Job drawing, mm, ordinate dimensions from the low corner. One solid piece. A direction names the side the tool comes from. Coordinates: 2 decimals unless noted, no trailing zeros. Write each loop counter-clockwise with the first axis right and the second up, starting at its lowest first coordinate (ties: lowest second). Pieces come first, ordered by that corner, then holes. Notation, with made-up numbers: (29, 43) - (83, 43) arc R12 cw to (83, 52) - close; hole circle Ø4 at (-16, 42). An arc over 180 degrees is marked (long way). Use one line per item in the form item = value. Start each with the question number.
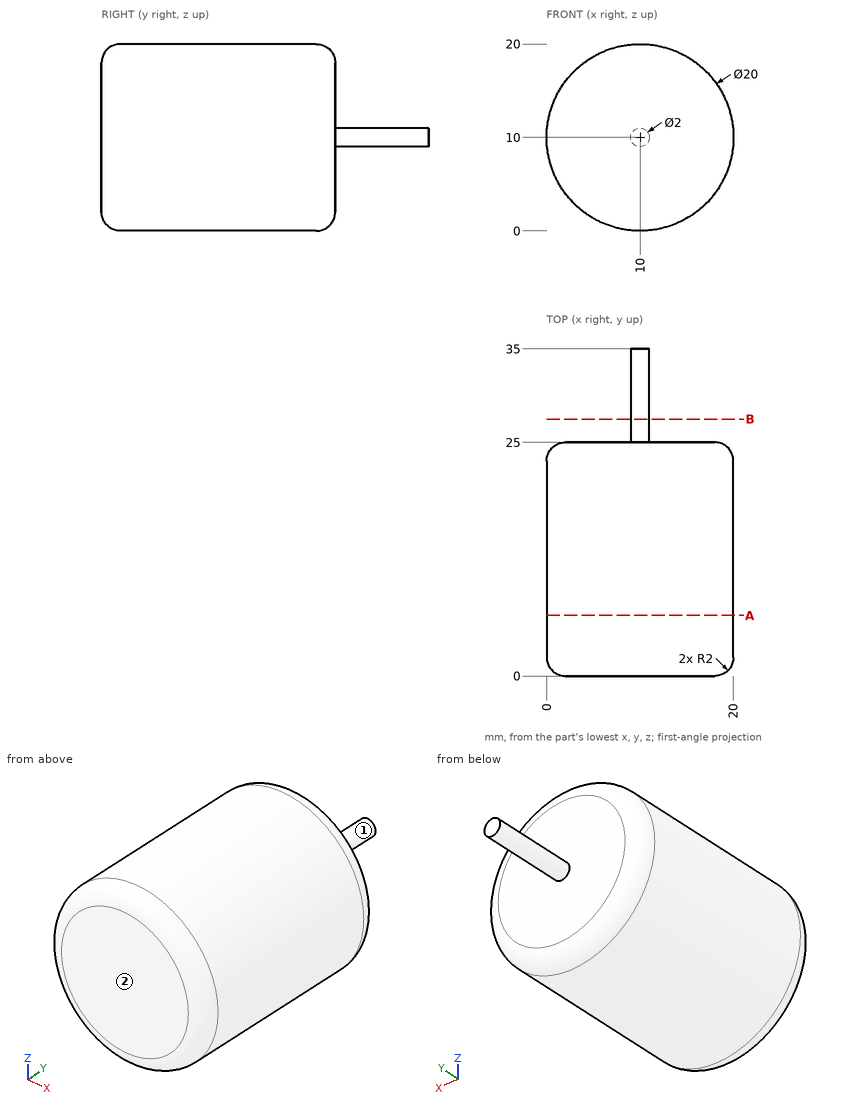
Q1. Which spindle directions (+Z, -Z, +X, -X, +Y, -Y) get a long thin tool onto all of the face, cutting with end or side? Do the marked faces 1 and 2. Say none if no direction does.
Q2. Pin check, flat tips, straight feed: P1, Ø12, axis at y = 15, z = 16.5, coming from the +X side; P2, Ø1.5, axis at x = 7.5, z = 7, coming from the +Y side; P3, Ø3, axis at y = 21.5, z = 5.5, coming from the -X side. Stop position of each tip, or through.
Q3. Drill centre lines: probe 1 along Y at (x, z) = (15, 4.25); probe 2 along X at (y, z) = (17, 16); probe 3 along Z at (x, y) = (10.25, 8.5). Where is each one in solid material? Low to high.
Q4. Slice it at A-A (y = 6.5). List the corners of the cut face in (x, z), plus the area to 3 significant figures.
Q5. Slice it at B-B (y = 27.5). List the corners of the cut face in (x, z).
Solution:
q1.face_1 = +Y
q1.face_2 = +Z, -Z, +X, -X, -Y
q2.P1 = 19.99
q2.P2 = 25
q2.P3 = 0.46
q3.probe_1 = 0 to 25
q3.probe_2 = 2 to 18
q3.probe_3 = 0 to 20
q4.outline = circle Ø20 at (10, 10)
q4.area = 314 mm2
q5.outline = circle Ø2 at (10, 10)
